```python
from build123d import *

# Parameters (mm, degrees)
SKETCH_W           = 8.94
SKETCH_H           = 3.16
PAD_DEPTH          = 3.95
SKETCH001_W        = 8.34
SKETCH001_H        = 2.56
POCKET_DEPTH       = 7.901
FILLET_R           = 1
FILLET001_R        = 1.3
CHAMFER_SIZE       = 0.15
SKETCH002_W        = 2
SKETCH002_H        = 1.9
SKETCH002_H_2      = 2.6
POCKET001_DEPTH    = 1.4
SKETCH003_W        = 0.3
SKETCH003_H        = 1.5
SKETCH003_H_2      = 1.3
PAD001_DEPTH       = 2
FILLET002_R        = 0.09
CHAMFER001_1_SIZE2 = 0.2
CHAMFER001_1_SIZE  = 0.5
CHAMFER001_2_SIZE2 = 0.2
CHAMFER001_2_SIZE  = 0.5
CHAMFER001_3_SIZE2 = 0.2
CHAMFER001_3_SIZE  = 0.5
CHAMFER002_SIZE2   = 0.5
CHAMFER002_SIZE    = 0.2
FILLET003_R        = 0.2
SKETCH004_W        = 5.8
SKETCH004_H        = 2.6
POCKET002_DEPTH    = 0.5
SKETCH005_W        = 1.7
SKETCH005_H        = 1.7
POCKET003_DEPTH    = 0.65
FILLET004_R        = 0.2


with BuildPart() as part:
    # Sketch → Pad (new body, symmetric)
    with BuildSketch(Plane.XZ):
        Rectangle(SKETCH_W, SKETCH_H)
    extrude(amount=PAD_DEPTH, both=True)

    # Sketch001 (on Face6 of Pad) → Pocket (cut, through all)
    with BuildSketch(Plane.XZ.offset(3.95)):
        Rectangle(SKETCH001_W, SKETCH001_H)
    extrude(amount=-POCKET_DEPTH, mode=Mode.SUBTRACT)

    # Fillet
    fillet_edges = [part.edges().sort_by_distance(p)[0] for p in [
        (-4.17, 0, -1.28),
        (-4.17, 0, 1.28),
        (4.17, 0, -1.28),
        (4.17, 0, 1.28),
    ]]
    fillet(fillet_edges, radius=FILLET_R)

    # Fillet001
    fillet001_edges = [part.edges().sort_by_distance(p)[0] for p in [
        (-4.47, 0, 1.58),
        (-4.47, 0, -1.58),
        (4.47, 0, 1.58),
        (4.47, 0, -1.58),
    ]]
    fillet(fillet001_edges, radius=FILLET001_R)

    # Chamfer
    chamfer_edges = [part.edges().sort_by_distance(p)[0] for p in [
        (0, -3.95, 1.28),
    ]]
    chamfer(chamfer_edges, length=CHAMFER_SIZE)

    # Sketch002 (on Face17 of Chamfer) → Pocket001 (cut)
    with BuildSketch(Plane(origin=(0, 0, -1.58), x_dir=(1, 0, 0), z_dir=(0, 0, -1))):
        with Locations((3.9, 1.25)):
            Rectangle(SKETCH002_W, SKETCH002_H)
        with Locations((-3.9, 1.25)):
            Rectangle(SKETCH002_W, SKETCH002_H)
        with Locations((-3.9, -2.65)):
            Rectangle(SKETCH002_W, SKETCH002_H_2)
        with Locations((3.9, -2.65)):
            Rectangle(SKETCH002_W, SKETCH002_H_2)
    extrude(amount=-POCKET001_DEPTH, mode=Mode.SUBTRACT)

    # Sketch003 (on Face5 of Pocket001) → Pad001 (join)
    with BuildSketch(Plane(origin=(0, 0, -0.18), x_dir=(1, 0, 0), z_dir=(0, 0, -1))):
        with Locations((-4.32, 1.25)):
            Rectangle(SKETCH003_W, SKETCH003_H)
        with Locations((4.32, 1.25)):
            Rectangle(SKETCH003_W, SKETCH003_H)
        with Locations((4.32, -3.3)):
            Rectangle(SKETCH003_W, SKETCH003_H_2)
        with Locations((-4.32, -3.3)):
            Rectangle(SKETCH003_W, SKETCH003_H_2)
    extrude(amount=PAD001_DEPTH)

    # Fillet002
    fillet002_edges = [part.edges().sort_by_distance(p)[0] for p in [
        (-4.32, -2, -0.18),
        (-4.32, -2.2, -0.18),
        (-4.32, -0.5, -0.18),
        (-4.32, -0.3, -0.18),
        (-4.32, 1.35, -0.18),
        (-4.32, 2.65, -0.18),
        (4.32, 2.65, -0.18),
        (4.32, 1.35, -0.18),
        (4.32, -2.2, -0.18),
        (4.32, -2, -0.18),
        (4.32, -0.5, -0.18),
        (4.32, -0.3, -0.18),
    ]]
    fillet(fillet002_edges, radius=FILLET002_R)

    # Chamfer001 1
    chamfer001_1_edges = [part.edges().sort_by_distance(p)[0] for p in [
        (4.32, -2, -2.18),
    ]]
    chamfer001_1_side = part.faces().sort_by_distance((4.32, -2, -1.225))[0]
    chamfer(chamfer001_1_edges, length=CHAMFER001_1_SIZE, length2=CHAMFER001_1_SIZE2, reference=chamfer001_1_side)

    # Chamfer001 2
    chamfer001_2_edges = [part.edges().sort_by_distance(p)[0] for p in [
        (4.32, -0.5, -2.18),
    ]]
    chamfer001_2_side = part.faces().sort_by_distance((4.32, -0.5, -1.225))[0]
    chamfer(chamfer001_2_edges, length=CHAMFER001_2_SIZE, length2=CHAMFER001_2_SIZE2, reference=chamfer001_2_side)

    # Chamfer001 3
    chamfer001_3_edges = [part.edges().sort_by_distance(p)[0] for p in [
        (-4.32, -2, -2.18),
    ]]
    chamfer001_3_side = part.faces().sort_by_distance((-4.32, -2, -1.225))[0]
    chamfer(chamfer001_3_edges, length=CHAMFER001_3_SIZE, length2=CHAMFER001_3_SIZE2, reference=chamfer001_3_side)

    # Chamfer002
    chamfer002_edges = [part.edges().sort_by_distance(p)[0] for p in [
        (-4.32, -0.5, -2.18),
    ]]
    chamfer002_side = part.faces().sort_by_distance((-4.32, -1.15, -2.18))[0]
    chamfer(chamfer002_edges, length=CHAMFER002_SIZE, length2=CHAMFER002_SIZE2, reference=chamfer002_side)

    # Fillet003
    fillet003_edges = [part.edges().sort_by_distance(p)[0] for p in [
        (-4.32, -0.7, -2.18),
        (-4.32, -1.8, -2.18),
        (-4.32, -0.5, -1.68),
        (-4.32, -2, -1.68),
        (4.32, -2, -1.68),
        (4.32, -0.5, -1.68),
        (4.32, -0.7, -2.18),
        (4.32, -1.8, -2.18),
        (4.32, 2.65, -2.18),
        (4.32, 3.95, -2.18),
        (-4.32, 2.65, -2.18),
        (-4.32, 3.95, -2.18),
    ]]
    fillet(fillet003_edges, radius=FILLET003_R)

    # Sketch004 (on Face36 of Fillet003) → Pocket002 (cut)
    with BuildSketch(Plane(origin=(0, 0, -1.58), x_dir=(1, 0, 0), z_dir=(0, 0, -1))):
        with Locations((0, -2.65)):
            Rectangle(SKETCH004_W, SKETCH004_H)
    extrude(amount=-POCKET002_DEPTH, mode=Mode.SUBTRACT)

    # Sketch005 (on Face24 of Pocket002) → Pocket003 (cut)
    with BuildSketch(Plane(origin=(0, 3.95, 0), x_dir=(1, 0, 0), z_dir=(0, 1, 0))):
        with Locations((-3.85, -1.05)):
            Rectangle(SKETCH005_W, SKETCH005_H)
        with Locations((3.85, -1.05)):
            Rectangle(SKETCH005_W, SKETCH005_H)
    extrude(amount=-POCKET003_DEPTH, mode=Mode.SUBTRACT)

    # Fillet004
    fillet004_edges = [part.edges().sort_by_distance(p)[0] for p in [
        (-3, 3.3, 1.43),
        (-4.32, 3.95, 0.2),
        (-4.32, 3.3, 0.2),
        (-3, 3.95, 1.43),
        (3, 3.95, 1.43),
        (3, 3.3, 1.43),
        (4.32, 3.3, 0.2),
        (4.32, 3.95, 0.2),
    ]]
    fillet(fillet004_edges, radius=FILLET004_R)


solid = part.part
```
Check sheet for the modelled part. Datum: model origin and axes. Units: mm. A direction names the side the tool comes from. Round coordinates to 2 decimals unless told otherwise and drop trailing zeros. Order: outer loops, then holes, each group sorted by start corner. A loop starts at its lowest first (then second) coordinate and runs counter-clockwise, first axis right, second up.
1) Mould release check, pull along Z, two halves, no side actions. Record for faces 1 (the cylindrical face through (3.869, 0.537, -0.995)), 2 (the flat face through (4.47, 1, 0)), 3 (the cylindrical face through (-4.1, -3.09, -1.19)), 4 (the cylindrical face through (4.08, -0.25, 1.21)): +Z half, -Z half, draft (parallel to the pull), parting line (faces both ways), or undercut.
2) Scan lines: line 1 (Z direction, x = 2.75, y = -1); line 2 (X direction, y = 2, z = 0.3); line 3 (Z direction, x = 1, y = 2.5). Record each from-to range of solid material in increasing order.
3) Tool access check on faces 5 (the cylindrical face through (-3.869, -2.989, -0.995)), 6 (the flat face through (4.17, 1, 0)), 7 (the cylindrical face through (-4.1, 0.51, -1.19)). Record the directions out of +Z, -Z, +X, -X, +Y, -Y that give a thin tool (end or side, any length) a straight path to the whole face; none if there is none.
4) Section check A-A (y = -3). Record the boundary of the cut face in (x, z).
5) Section check C-C (z = -0.9). Give the number of separate pieces and of enclosed holes in the cut face, and give its area (3 significant figures).
6) Go/stop test with a flat-tipped pin: pin 1 Ø1 at (x, z) = (-0.5, -1) entering from +Y. Record where the tip stops, or that it passes through.
7) Section check B-B (x = 0). Record the boundary of the cut face in (y, z).
Result:
1. face 1: undercut
1. face 2: draft
1. face 3: -Z half
1. face 4: +Z half
2. line 1: z = -1.58 to -1.28, 1.28 to 1.58
2. line 2: x = -4.47 to -4.17, 4.17 to 4.47
2. line 3: z = 1.28 to 1.58
3. face 5: +Y, -Y
3. face 6: none
3. face 7: -Z, -X
4. outline: (-4.47, -0.28) arc R1.3 ccw to (-3.17, -1.58) - (3.17, -1.58) arc R1.3 ccw to (4.47, -0.28) - (4.47, 0.28) arc R1.3 ccw to (3.17, 1.58) - (-3.17, 1.58) arc R1.3 ccw to (-4.47, 0.28) - close; hole (-4.17, -0.28) arc R1 ccw to (-3.17, -1.28) - (3.17, -1.28) arc R1 ccw to (4.17, -0.28) - (4.17, 0.28) arc R1 ccw to (3.17, 1.28) - (-3.17, 1.28) arc R1 ccw to (-4.17, 0.28) - close
5. separate pieces: 8
5. enclosed holes: 0
5. area: 4.09 mm2
6. pin 1: stops at y = 1.35
7. outline: (-3.95, -1.58) - (1.35, -1.58) - (1.35, -1.28) - (-3.8, -1.28) - (-3.95, -1.43) - close; (-3.95, 1.43) - (-3.8, 1.28) - (3.95, 1.28) - (3.95, 1.58) - (-3.95, 1.58) - close
